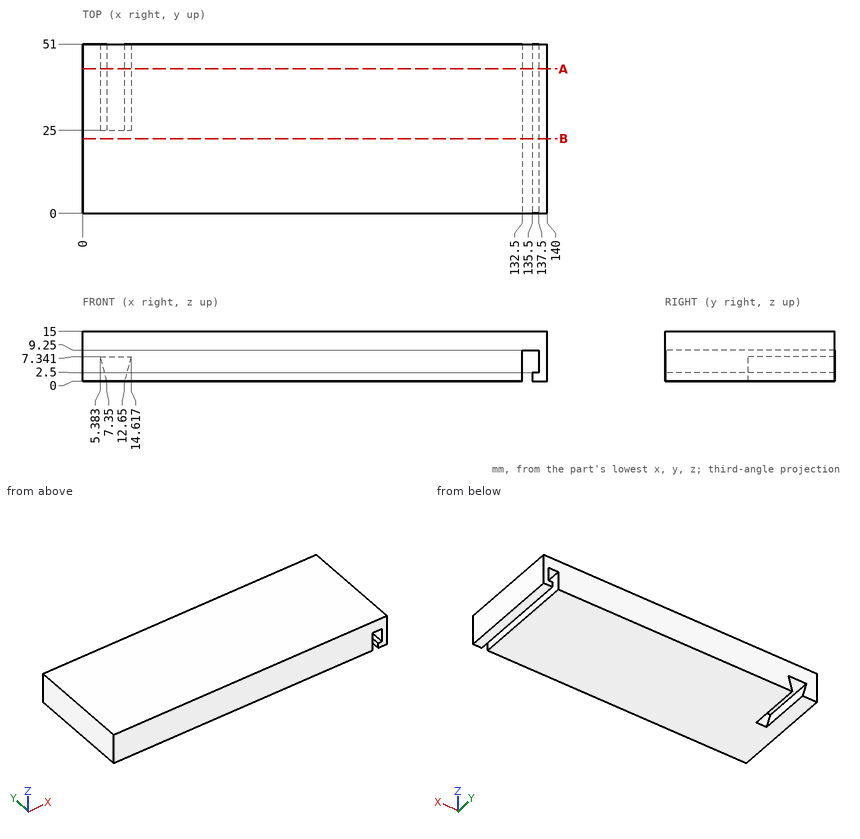
Could you check a few things on this drawing? It's one solid part, dimensions in mm from its lowest x, y, z. Coordinates: 2 decimals unless noted, no trailing zeros. Loops run counter-clockwise (first coordinate to the right, second up) from the corner with the lowest first, then second, coordinate; pieces in that order, holes last. Notation, with made-up numbers: (-7, 72) - (32, 72) arc R37 ccw to (32, 108) - close; hole circle Ø10 at (68.25, 14.25). An arc over 180 degrees is marked (long way). Return JSON: item names as keys, results as strings. Group by question number.
Item 1: If we section it at B-B on y = 22.5: Write out the boundary of the cut face in (x, z), and give its area (3 significant figures).
Item 2: I need wall thicknesses on line 1 (X direction, y = 49, z = 1); line 2 (X direction, y = 37.5, z = 2). Which ranges of each line are inside material? Lowest first, please. Write a range as from..to.
Item 3: Will these pins go through, and if not, where does the flat tip stop? P1, Ø3.5, axis at x = 10.5, z = 2.5, coming from the +Y side; P2, Ø1.5, axis at x = 134.5, y = 28, coming from the -Z side.
Item 4: If we section it at A-A on y = 43.5: Write out the boundary of the cut face in (x, z).
Calculated:
{
 "1": {"outline": "(0, 0) - (132.5, 0) - (132.5, 9.25) - (137.5, 9.25) - (137.5, 2.5) - (135.5, 2.5) - (135.5, 0) - (140, 0) - (140, 15) - (0, 15) - close", "area": "2,060 mm^2"},
 "2": {"line 1": "x = 0..7.08, 12.92..132.5, 135.5..140", "line 2": "x = 0..6.81, 13.19..132.5, 135.5..140"},
 "3": {"P1": "stops at y = 25", "P2": "stops at z = 9.25"},
 "4": {"outline": "(0, 0) - (7.35, 0) - (5.38, 7.34) - (14.62, 7.34) - (12.65, 0) - (132.5, 0) - (132.5, 9.25) - (137.5, 9.25) - (137.5, 2.5) - (135.5, 2.5) - (135.5, 0) - (140, 0) - (140, 15) - (0, 15) - close"}
}
